from build123d import *

# Parameters (mm, degrees)
BOSS_EXTRUDE1_DEPTH      = 50
BOSS_EXTRUDE2_START      = 5
BOSS_EXTRUDE2_DEPTH      = 5
SKETCH3_R                = 15
BOSS_EXTRUDE3_DEPTH      = 3
FILLET1_R                = 3
M16X1_5_TAPPED_HOLE1_D   = 14.5
BOSS_EXTRUDE6_REACH      = 120.042
BOSS_EXTRUDE6_END_RADIUS = 50
SKETCH11_R               = 15
M10X1_0_TAPPED_HOLE1_D   = 9
SKETCH15_R               = 8
CUT_EXTRUDE1_DEPTH       = 114.903467988
FILLET2_R                = 2
FILLET3_R                = 4


with BuildPart() as part:
    # Sketch1 → Boss-Extrude1 (new, symmetric)
    with BuildSketch(Plane.XY):
        with BuildLine():
            Line((-40, 0), (-45, 0))
            Line((-45, 0), (-45, 5))
            Line((-45, 5), (-90, 5))
            Line((-90, 5), (-90, 25))
            Line((-90, 25), (-43.301270189, 25))
            ThreePointArc((-43.301270189, 25), (0, 50), (43.301270189, 25))
            Line((43.301270189, 25), (90, 25))
            Line((90, 25), (90, 5))
            Line((90, 5), (45, 5))
            Line((45, 5), (45, 0))
            Line((45, 0), (40, 0))
            ThreePointArc((40, 0), (0, 40), (-40, 0))
        make_face()
    extrude(amount=BOSS_EXTRUDE1_DEPTH, both=True)

    # Sketch2 → Boss-Extrude2 (add)
    with BuildSketch(Plane.XY.offset(50).offset(BOSS_EXTRUDE2_START)):
        with BuildLine():
            Line((40, 0), (45, 0))
            Line((45, 0), (45, 5))
            Line((45, 5), (49.749371855, 5))
            ThreePointArc((49.749371855, 5), (0, 50), (-49.749371855, 5))
            Line((-49.749371855, 5), (-45, 5))
            Line((-45, 5), (-45, 0))
            Line((-45, 0), (-40, 0))
            ThreePointArc((-40, 0), (0, 40), (40, 0))
        make_face()
    boss_extrude2 = extrude(amount=-BOSS_EXTRUDE2_DEPTH)

    # Mirror1: Boss-Extrude2 across plane
    add(boss_extrude2.mirror(Plane.XY))

    # Sketch3 → Boss-Extrude3 (add)
    with BuildSketch(Plane(origin=(0, 25, 0), x_dir=(1, 0, 0), z_dir=(0, 1, 0))):
        with Locations(Location((-70, 0, 0), (0, 0, 270))):
            Circle(SKETCH3_R)
        with Locations(Location((70, 0, 0), (0, 0, 270))):
            Circle(SKETCH3_R)
    extrude(amount=BOSS_EXTRUDE3_DEPTH)

    # Fillet1
    fillet1_edges = [part.edges().sort_by_distance(p)[0] for p in [
        (-70, 25, -15),
        (70, 25, -15),
    ]]
    fillet(fillet1_edges, radius=FILLET1_R - 0.0001)  # a hair under: the kernel refuses the full size

    # M16x1.5 Tapped Hole1 (through all)
    with Locations(Plane(origin=(0, 28, 0), x_dir=(1, 0, 0), z_dir=(0, 1, 0))):
        with Locations((-70, 0), (70, 0)):
            Hole(M16X1_5_TAPPED_HOLE1_D / 2)

    # Boss-Extrude6: up to this cylinder (the profile starts outside it)
    boss_extrude6_end = Plane(origin=(0, 0, 0), z_dir=(0, 0, 1)) * Cylinder(BOSS_EXTRUDE6_END_RADIUS, 341.084, mode=Mode.PRIVATE)
    # Sketch11 → Boss-Extrude6 (add, up to the surface)
    with BuildSketch(Plane(origin=(0, 53, 0), x_dir=(-1, 0, 0), z_dir=(0, -1, 0)), mode=Mode.PRIVATE) as boss_extrude6_sk1:
        Circle(SKETCH11_R)
    boss_extrude6_tool1 = extrude(boss_extrude6_sk1.sketch, amount=BOSS_EXTRUDE6_REACH, mode=Mode.PRIVATE) - boss_extrude6_end
    add(boss_extrude6_tool1.solids().sort_by_distance((0, 53, 0))[0])

    # M10x1.0 Tapped Hole1 (through all)
    with Locations(Plane(origin=(0, 53, 0), x_dir=(1, 0, 0), z_dir=(0, 1, 0))):
        with Locations((0, 0)):
            Hole(M10X1_0_TAPPED_HOLE1_D / 2)

    # Sketch15 → Cut-Extrude1 (cut, through all)
    with BuildSketch(Plane(origin=(0, 43, 0), x_dir=(-1, 0, 0), z_dir=(0, -1, 0))):
        Circle(SKETCH15_R)
    extrude(amount=CUT_EXTRUDE1_DEPTH, mode=Mode.SUBTRACT)

    # Fillet2
    fillet2_edges = [part.edges().sort_by_distance(p)[0] for p in [
        (-43.301270189, 25, 0),
        (43.301270189, 25, 0),
    ]]
    fillet(fillet2_edges, radius=FILLET2_R)

    # Fillet3
    fillet3_edges = [part.edges().sort_by_distance(p)[0] for p in [
        (-90, 15, 50),
        (90, 15, 50),
        (90, 15, -50),
        (-90, 15, -50),
    ]]
    fillet(fillet3_edges, radius=FILLET3_R)


solid = part.part
For this review, take the finished solid that the model builds, in its own axes (mm). A direction names the side the tool comes from. Round coordinates to 2 decimals unless told otherwise and drop trailing zeros. Write each loop counter-clockwise with the first axis right and the second up, starting at its lowest first coordinate (ties: lowest second). Pieces come first, ordered by that corner, then holes. Notation, with made-up numbers: M 1,69 L 35,69 A26 cw 35,86 Z; hole C 0.25,42 d9. An arc over 180 degrees is marked long. Write item = value, one per line. Start each with the question number.
(1) We need section C-C (z = -24). Give the boundary of the cut face in (x, y).
(2) For faces 1 (the face through (90, 15, 1)), 2 (the face through (-58, 5, -1)), 3 (the face through (-7.39, 41.12, 3.06)), list the 3-axis set-ups (+Z, -Z, +X, -X, +Y, -Y) from which the entire face can be reached by the end or side of a thin tool; tool diameter is ignored.
(3) The part is to be moulded in two halves that separate along Z. For faces 4 (the face through (-3.4, 43, 3.4)), 5 (the face through (65, 16, -50)), 6 (the face through (-90, 15, 1)), 7 (the face through (-88.859, 15.14, 48.797)), say which applies: +Z half, -Z half, draft (parallel to the pull), parting line (faces both ways), or undercut.
(4) We need section B-B (y = 23). Give the boundary of the cut face in (x, z), then the cut area to 3 significant figures.
(5) For line 1 along Z through (x, y) = (-70, 10); line 2 along Z through (x, y) = (0, 48.5); line 3 along Y through (x, z) = (55.5, 1.5), list the stretches that pass through material, from the lowest coordinate up.
(6) Clearance check with flat-ended pins moving along their axes: pin 1 Ø8 at (x, z) = (0, 0) entering from -Y; pin 2 Ø22.5 at (x, z) = (-76, -10) entering from -Y; pin 3 Ø1.5 at (y, z) = (44, 40.5) entering from -X; pin 4 Ø4 at (x, z) = (6.5, 43) entering from -Y. State where each tip first meets the part, or that it passes through.
(7) We need section D-D (y = 7). Give the boundary of the cut face in (x, z).
Results found:
q1.outline = M -90,5 L -45,5 L -45,0 L -40,0 A40 cw 40,0 L 45,0 L 45,5 L 90,5 L 90,25 L 44.44,25 A2 cw 42.73,25.96 A50 ccw -42.73,25.96 A2 cw -44.44,25 L -90,25 Z
q2.face_1 = +Z, -Z, +X, +Y, -Y
q2.face_2 = +Z, -Z, -X, -Y
q2.face_3 = -Y
q3.face_4 = undercut
q3.face_5 = -Z half
q3.face_6 = draft
q3.face_7 = +Z half
q4.outline = M -90,-46 A4 ccw -86,-50 L -44.4,-50 L -44.4,-55 L -32.73,-55 L -32.73,55 L -44.4,55 L -44.4,50 L -86,50 A4 ccw -90,46 Z; M 32.73,-55 L 44.4,-55 L 44.4,-50 L 86,-50 A4 ccw 90,-46 L 90,46 A4 ccw 86,50 L 44.4,50 L 44.4,55 L 32.73,55 Z; hole C -70,0 d14.5; hole C 70,0 d14.5
q4.area = 11,300 mm²
q5.line_1 = -50 to -7.25, 7.25 to 50
q5.line_2 = -55 to -4.5, 4.5 to 55
q5.line_3 = 5 to 28
q6.pin_1 = through
q6.pin_2 = 5
q6.pin_3 = -25.09
q6.pin_4 = 39.09
q7.outline = M -90,-46 A4 ccw -86,-50 L -49.51,-50 L -49.51,-55 L -39.38,-55 L -39.38,55 L -49.51,55 L -49.51,50 L -86,50 A4 ccw -90,46 Z; M 39.38,-55 L 49.51,-55 L 49.51,-50 L 86,-50 A4 ccw 90,-46 L 90,46 A4 ccw 86,50 L 49.51,50 L 49.51,55 L 39.38,55 Z; hole C -70,0 d14.5; hole C 70,0 d14.5
